Geometry check sheet. Reference: drawing and pictorial views, mm from the part's lowest x, y, z. A direction names the side the tool comes from. Round coordinates to 2 decimals unless told otherwise and drop trailing zeros. Loops run counter-clockwise (first coordinate to the right, second up) from the corner with the lowest first, then second, coordinate; pieces in that order, holes last. Notation, with made-up numbers: (-36.75, 25.5) -> (-28.75, 25.5) arc R25 cw to (-28.75, 61.5) -> close; hole circle Ø3 at (57, 55.25). An arc over 180 degrees is marked (long way). Use one line per item in the form item = value. Start each with the question number.
(1) Sectioned sample at B-B (z = 58). Record the cut outline in (x, y), and give its area (3 significant figures).
(2) Set-up check for the marked faces 1, 2, 3, 4 and 5: record each of +Z, -Z, +X, -X, +Y, -Y from which the full face is reachable in a straight line by a thin tool's end or side.
(3) Material ranges on probe 1 along X at (y, z) = (43.5, 64); probe 2 along Z at (x, y) = (44, 37); probe 3 along Z at (x, y) = (13, 7.5), recorded low to high. Write a range as [from, to].
(4) Sectioned sample at A-A (x = 70.5). Record the cut outline in (y, z).
(5) Go/stop test with flat-tipped pins: pin 1 (12 mm diameter, centred on x = 35.5, y = 36, fed in from -Z); pin 2 (10 mm diameter, centred on x = 12.5, y = 22.5, fed in from +Z); pin 3 (1.6 mm diameter, centred on x = 45.5, y = 1, fed in from +Z). Record where each tip stops, or that it passes through.
(6) Sectioned sample at D-D (x = 58). Record the cut outline in (y, z), and give its area (3 significant figures).
(7) Sectioned sample at C-C (y = 45). Record the cut outline in (x, z).
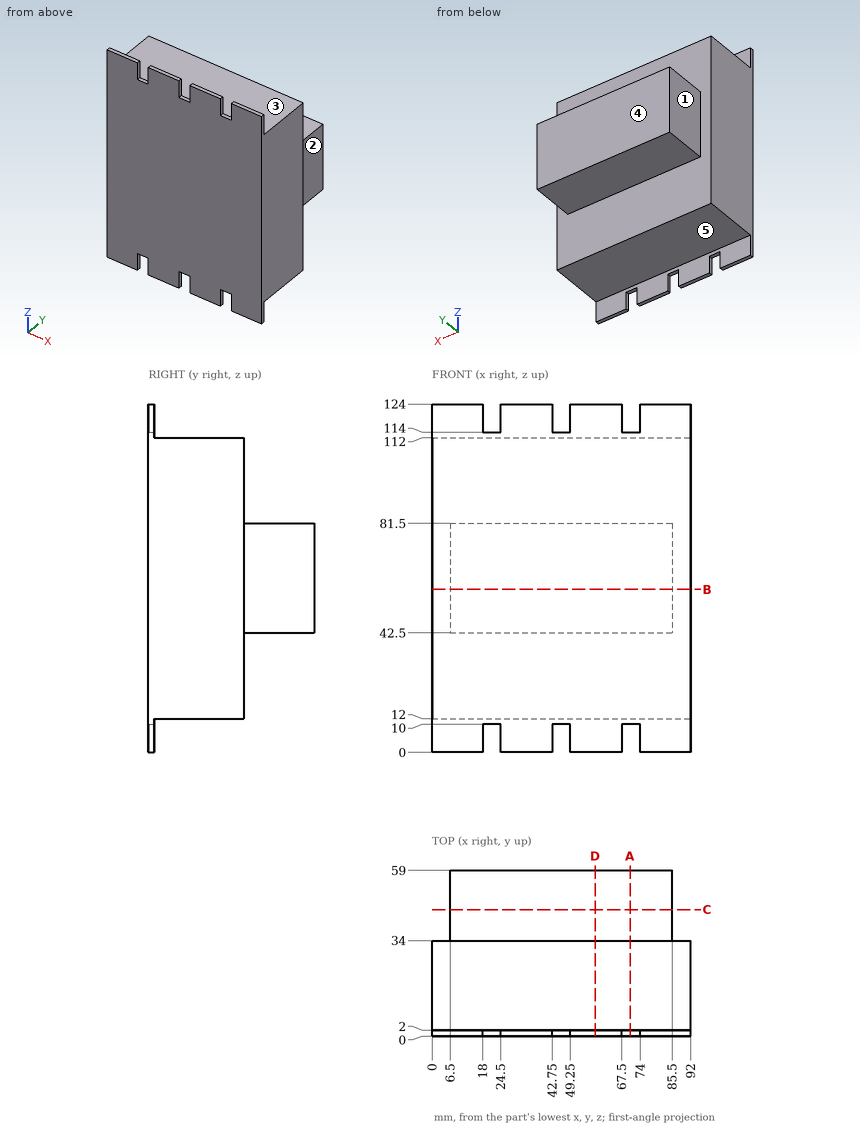
Checks:
q1.outline = (0, 0) -> (92, 0) -> (92, 34) -> (85.5, 34) -> (85.5, 59) -> (6.5, 59) -> (6.5, 34) -> (0, 34) -> close
q1.area = 5,100 mm2
q2.face_1 = +Z, -Z, -X, +Y
q2.face_2 = +Z, -Z, +X, +Y
q2.face_3 = +Z, +X, -X, +Y
q2.face_4 = +Z, -Z, +X, -X, +Y
q2.face_5 = -Z, +X, -X, +Y
q3.probe_1 = [6.5, 85.5]
q3.probe_2 = [42.5, 81.5]
q3.probe_3 = [12, 112]
q4.outline = (0, 10) -> (2, 10) -> (2, 12) -> (34, 12) -> (34, 42.5) -> (59, 42.5) -> (59, 81.5) -> (34, 81.5) -> (34, 112) -> (2, 112) -> (2, 114) -> (0, 114) -> close
q5.pin_1 = 12
q5.pin_2 = 112
q5.pin_3 = 114
q6.outline = (0, 0) -> (2, 0) -> (2, 12) -> (34, 12) -> (34, 42.5) -> (59, 42.5) -> (59, 81.5) -> (34, 81.5) -> (34, 112) -> (2, 112) -> (2, 124) -> (0, 124) -> close
q6.area = 4,420 mm2
q7.outline = (6.5, 42.5) -> (85.5, 42.5) -> (85.5, 81.5) -> (6.5, 81.5) -> close
